Input: part model. Units: mm. Frame: model coordinates. A direction names the side the tool comes from. Coordinates: 2 decimals unless noted, no trailing zeros. Write each loop counter-clockwise with the first axis right and the second up, starting at its lowest first coordinate (ties: lowest second). Pieces come first, ordered by that corner, then holes. Notation, with made-up numbers: (81, 49) -> (122, 49) arc R26 cw to (122, 68) -> close; hole circle Ø10 at (0, -31). An arc over 180 degrees is marked (long way). Use one line per item in the form item = value. Start each with the question number.
(1) Cut plane A-A on z = 24. Return the cut outline in (x, y).
(2) Cut plane C-C on x = -21.5. Return the cut outline in (y, z), plus the area to 3 significant figures.
(3) Set-up query: faces 1 (the face through (-6.845, -2.789, 23.451)), 2 (the face through (23, -2, 3)), 3 (the face through (-13.221, -0.14, 0.593)), 4 (the face through (2.9, 6.8, 23.5)). Return all of +Z, -Z, +X, -X, +Y, -Y with unobstructed straight access to the full face (end or side cutting, diameter ignored); none if empty.
(4) Cut plane D-D on z = 13.25. Return the cut outline in (x, y), plus the area to 3 significant figures.
(5) Cut plane B-B on x = 24.92. Return the cut outline in (y, z), plus the area to 3 significant figures.
(6) Ray query, line 1 along Y through (x, z) = (24.92, 1.65); line 2 along Y through (x, z) = (0, 23.5); line 3 along Z through (x, y) = (-24, -8). Return the intervals inside material, ascending.
(7) First-contact query: pin 1 (10.5 mm diameter, centred on x = 0, y = 0, fed in from -Z); pin 2 (9 mm diameter, centred on x = 21, y = 4.5, fed in from +Z); pin 3 (6 mm diameter, centred on y = -2, z = 14.5, fed in from -X). Flat tips, straight axial feed; report the tip coordinate or a pass-through.
(8) Pull-direction query (X, two-part tool) for faces 5 (the face through (0, 0, 16)), 6 (the face through (-8.27, -0.14, 14.44)), 7 (the face through (-5, -2, 18)); classes: released by +X, released by -X, zero draft, split by the parting line, or undercut.
```python
from build123d import *

# Parameters (mm, degrees)
F1_DEPTH  = 10
F2_R      = 2.5
F3_DEPTH  = 25
F5_DEPTH  = 3
F7_DEPTH  = 3
F8_R      = 5
F9_DEPTH  = 2
F11_DEPTH = 7
F12_R     = 5
F12_R_2   = 4
F13_DEPTH = 1.5
F14_DEPTH = 11


with BuildPart() as f1:
    # F0 (on Front) → F1 (new body, symmetric)
    with BuildSketch(Plane.XZ):
        with BuildLine():
            ThreePointArc((-7, 18), (-8.2975682269, 14.3901805601), (-10.5921510788, 11.3161979271))
            ThreePointArc((-10.5921510788, 11.3161979271), (-13.3053586993, 7.950938931), (-14.9836855606, 3.9672619048))
            ThreePointArc((-14.9836855606, 3.9672619048), (-15.4474629596, 3.2698156661), (-16.2403817689, 3))
            Line((-16.2403817689, 3), (-29.85, 3))
            Line((-29.85, 3), (-29.85, 0))
            Line((-29.85, 0), (-14.8744747806, 0))
            ThreePointArc((-14.8744747806, 0), (-13.2017484895, 0.6095259974), (-12.3133069376, 2.1523178808))
            ThreePointArc((-12.3133069376, 2.1523178808), (0, 12.5), (12.3133069376, 2.1523178808))
            ThreePointArc((12.3133069376, 2.1523178808), (13.2017484895, 0.6095259974), (14.8744747806, 0))
            Line((14.8744747806, 0), (29.85, 0))
            Line((29.85, 0), (29.85, 3))
            Line((29.85, 3), (16.2403817689, 3))
            ThreePointArc((16.2403817689, 3), (15.4474629596, 3.2698156661), (14.9836855606, 3.9672619048))
            ThreePointArc((14.9836855606, 3.9672619048), (13.3053586993, 7.950938931), (10.5921510788, 11.3161979271))
            ThreePointArc((10.5921510788, 11.3161979271), (8.2975682269, 14.3901805601), (7, 18))
            Line((7, 18), (-7, 18))
        make_face()
    extrude(amount=F1_DEPTH, both=True)

    # F2 (on face) → F3 (cut)
    with BuildSketch(Plane.XY.offset(3)):
        with Locations((-24.92, 0)):
            Circle(F2_R)
        with Locations((24.92, 0)):
            Circle(F2_R)
    extrude(amount=-F3_DEPTH, mode=Mode.SUBTRACT)

    # F4 (on face) → F5 (join, through all)
    with BuildSketch(Plane.XY.offset(3)):
        with BuildLine():
            Line((-29.85, -10), (-29.85, 10))
            ThreePointArc((-29.85, 10), (-33.7754930507, 0), (-29.85, -10))
        make_face()
    extrude(amount=-F5_DEPTH)

    # F6 (on face) → F7 (join, through all)
    with BuildSketch(Plane.XY.offset(3)):
        with BuildLine():
            Line((29.85, 10), (29.85, -10))
            ThreePointArc((29.85, -10), (33.7754930507, 0), (29.85, 10))
        make_face()
    extrude(amount=-F7_DEPTH)

    # F8 (on face) → F9 (join)
    with BuildSketch(Plane.XY.offset(18)):
        Circle(F8_R)
    extrude(amount=F9_DEPTH)

    # F10 (on face) → F11 (join)
    with BuildSketch(Plane.XY.offset(20)):
        Polygon((-5.6568542495, -5.6568542495), (0, -8), (5.6568542495, -5.6568542495), (8, 0), (5.6568542495, 5.6568542495), (0, 8), (-5.6568542495, 5.6568542495), (-8, 0), align=None)
    extrude(amount=F11_DEPTH)

    # F12 (on face) → F13 (join)
    with BuildSketch(Plane.XY.offset(27)):
        Circle(F12_R)
        Circle(F12_R_2, mode=Mode.SUBTRACT)
    extrude(amount=F13_DEPTH)

    # F14 (cut): a face of the model
    f14_faces = [f1.faces().sort_by_distance(p)[0] for p in [
        (0, 0, 27),
    ]]
    extrude(f14_faces, amount=-F14_DEPTH, mode=Mode.SUBTRACT)


solid = f1.part
```
Values:
q1.outline = (-8, 0) -> (-5.66, -5.66) -> (0, -8) -> (5.66, -5.66) -> (8, 0) -> (5.66, 5.66) -> (0, 8) -> (-5.66, 5.66) -> close; hole circle Ø8 at (0, 0)
q2.outline = (-10, 0) -> (10, 0) -> (10, 3) -> (-10, 3) -> close
q2.area = 60.0 mm2
q3.face_1 = +Z, -X, -Y
q3.face_2 = +Z, +X, +Y, -Y
q3.face_3 = -Z, +Y, -Y
q3.face_4 = +Z, +X, +Y
q4.outline = (-8.99, -10) -> (8.99, -10) -> (8.99, 10) -> (-8.99, 10) -> close
q4.area = 360 mm2
q5.outline = (-10, 0) -> (-2.5, 0) -> (-2.5, 3) -> (-10, 3) -> close; (2.5, 0) -> (10, 0) -> (10, 3) -> (2.5, 3) -> close
q5.area = 45.0 mm2
q6.line_1 = -10 to -2.5, 2.5 to 10
q6.line_2 = -8 to -4, 4 to 8
q6.line_3 = 0 to 3
q7.pin_1 = 11.34
q7.pin_2 = 3
q7.pin_3 = -10.41
q8.face_5 = undercut
q8.face_6 = released by -X
q8.face_7 = zero draft
